from build123d import *

# Parameters (mm, degrees)
SKETCH1_R                                       = 152.5
SKETCH1_R_2                                     = 137.5
BOSS_EXTRUDE1_DEPTH                             = 14.4
CSK_FOR_M5_FLAT_HEAD_MACHINE_SCREW1_D           = 5.5
CSK_FOR_M5_FLAT_HEAD_MACHINE_SCREW1_CSINK_D     = 10.4
CSK_FOR_M5_FLAT_HEAD_MACHINE_SCREW1_CSINK_ANGLE = 90
CIRPATTERN1_COUNT                               = 6


with BuildPart() as part:
    # Sketch1 → Boss-Extrude1 (new body)
    with BuildSketch(Plane(origin=(0, 0, 0), x_dir=(1, 0, 0), z_dir=(0, 1, 0))):
        with Locations(Location((0, 0, 0), (0, 0, 270))):
            Circle(SKETCH1_R)
        with Locations(Location((0, 0, 0), (0, 0, 270))):
            Circle(SKETCH1_R_2, mode=Mode.SUBTRACT)
    extrude(amount=BOSS_EXTRUDE1_DEPTH)

    # CSK for M5 Flat Head Machine Screw1 (through all)
    with Locations(Plane(origin=(0, 14.4, 0), x_dir=(1, 0, 0), z_dir=(0, 1, 0))):
        with Locations((0, 146.25)):
            csk_for_m5_flat_head_machine_screw1 = CounterSinkHole(CSK_FOR_M5_FLAT_HEAD_MACHINE_SCREW1_D / 2, CSK_FOR_M5_FLAT_HEAD_MACHINE_SCREW1_CSINK_D / 2, counter_sink_angle=CSK_FOR_M5_FLAT_HEAD_MACHINE_SCREW1_CSINK_ANGLE)

    # CirPattern1: CSK for M5 Flat Head Machine Screw1 ×6 about axis
    cirpattern1_axis = Axis((0, 0, 0), (0, 1, 0))
    for i in range(1, CIRPATTERN1_COUNT):
        add(csk_for_m5_flat_head_machine_screw1.rotate(cirpattern1_axis, i * 360 / CIRPATTERN1_COUNT), mode=Mode.SUBTRACT)


solid = part.part
The listing builds one solid part. Answer for the finished solid, in the listing's coordinates (mm). Round coordinates to 2 decimals unless told otherwise and drop trailing zeros. Order: outer loops, then holes, each group sorted by start corner. A loop starts at its lowest first (then second) coordinate and runs counter-clockwise, first axis right, second up. Notation, with made-up numbers: (18.25, -26.75) -> (39.25, -26.75) arc R37 cw to (39.25, 9.25) -> close; hole circle Ø10 at (69.25, 22). An arc over 180 degrees is marked (long way). Write each question's results on one line, items separated by ' | '. Start each with the question number.
Q1. Each of these flat-tipped pins is pushed along its axis until it touches: pin 1 (3.5 mm diameter, centred on x = 0, z = 146.25, fed in from +Y); pin 2 (4 mm diameter, centred on y = 5, z = 54.5, fed in from -X); pin 3 (4 mm diameter, centred on y = 9, z = -69.5, fed in from -X); pin 4 (6.5 mm diameter, centred on x = -126.66, z = 73.12, fed in from +Y). Where does it stop, or does it pass through?
Q2. Straight lines are drawn through the part: probe 1 along X at (y, z) = (5.5, 2.5); probe 2 along Z at (x, y) = (116.5, 11.75); probe 3 along Z at (x, y) = (-9.5, 11.25). For each, find the intervals that lie inside material, in ascending order. Write a range as from..to.
Q3. Find section C-C (y = 4). Determine the outline of the cut face in (x, z) (3 decimals), then the cut area to 3 significant figures.
Q4. Find section A-A (z = 0). Determine the outline of the cut face in (x, y), then the cut area to 3 significant figures.
Q5. Find section B-B (x = -104.5). Determine the outline of the cut face in (y, z).
Q6. The mould has two halves that part along Z. Classify faces 1 (the conical face through (-127.03, 12.07, -70.28)), 2 (the cylindrical face through (45.807, 7.099, 145.458)), 3 (the flat face through (-112.3, 14.4, -79.8)): pulls with the +Z half, pulls with the -Z half, needs draft (parallel to the pull), parting line crosses it, or undercut.
Worked answers:
1) pin 1: passes through | pin 2: stops at x = -143.18 | pin 3: stops at x = -136.75 | pin 4: stops at y = 12.46
2) probe 1: x = -152.48..-137.48, 137.48..152.48 | probe 2: z = -98.41..-73.03, 73.03..98.41 | probe 3: z = -152.2..-137.17, 137.17..152.2
3) outline: circle Ø305 at (0, 0); hole circle Ø275 at (0, 0); hole circle Ø5.5 at (-126.656, -73.125); hole circle Ø5.5 at (-126.656, 73.125); hole circle Ø5.5 at (0, -146.25); hole circle Ø5.5 at (0, 146.25); hole circle Ø5.5 at (126.656, -73.125); hole circle Ø5.5 at (126.656, 73.125) | area: 13,500 mm2
4) outline: (-152.5, 0) -> (-137.5, 0) -> (-137.5, 14.4) -> (-152.5, 14.4) -> close; (137.5, 0) -> (152.5, 0) -> (152.5, 14.4) -> (137.5, 14.4) -> close | area: 432 mm2
5) outline: (0, -111.07) -> (14.4, -111.07) -> (14.4, -89.36) -> (0, -89.36) -> close; (0, 89.36) -> (14.4, 89.36) -> (14.4, 111.07) -> (0, 111.07) -> close
6) face 1: undercut | face 2: parting line crosses it | face 3: needs draft
